from build123d import *

# Parameters (mm, degrees)
SKETCH_1_W          = 54
SKETCH_1_H          = 15
SKETCH_1_R          = 2.75
EXTRUDE_1_DEPTH     = 6
SKETCH_2_W          = 15
SKETCH_2_H          = 35
EXTRUDE_2_DEPTH     = 7.5
SKETCH_3_R          = 2.25
CUT_EXTRUDE_1_DEPTH = 15
CHAMFER_1_SIZE      = 2
FILLET_1_R          = 1


with BuildPart() as part:
    # 草图1 → 凸台-拉伸1 (new body)
    with BuildSketch(Plane(origin=(0, 0, 0), x_dir=(1, 0, 0), z_dir=(0, 1, 0))):
        Rectangle(SKETCH_1_W, SKETCH_1_H)
        with Locations(Location((-20, 0, 0), (0, 0, 270))):
            Circle(SKETCH_1_R, mode=Mode.SUBTRACT)
        with Locations(Location((20, 0, 0), (0, 0, 270))):
            Circle(SKETCH_1_R, mode=Mode.SUBTRACT)
    extrude(amount=EXTRUDE_1_DEPTH)

    # 草图2 → 凸台-拉伸2 (add, symmetric)
    with BuildSketch(Plane.XY):
        with Locations((0, 23.5)):
            Rectangle(SKETCH_2_W, SKETCH_2_H)
    extrude(amount=EXTRUDE_2_DEPTH, both=True)

    # 草图3 → 切除-拉伸1 (cut)
    with BuildSketch(Plane.ZY.offset(7.5)):
        with Locations(Location((0, 11, 0), (0, 0, 270))):
            Circle(SKETCH_3_R)
        with Locations(Location((0, 37, 0), (0, 0, 270))):
            Circle(SKETCH_3_R)
    extrude(amount=-CUT_EXTRUDE_1_DEPTH, mode=Mode.SUBTRACT)

    # 倒角1
    chamfer_1_edges = [part.edges().sort_by_distance(p)[0] for p in [
        (7.5, 6, 0),
        (-7.5, 6, 0),
    ]]
    chamfer(chamfer_1_edges, length=CHAMFER_1_SIZE)

    # 圆角1
    fillet_1_edges = [part.edges().sort_by_distance(p)[0] for p in [
        (-27, 6, 0),
        (-18.25, 6, 7.5),
        (0, 41, -7.5),
        (7.5, 41, 0),
        (-7.5, 24.5, -7.5),
        (-7.5, 41, 0),
        (0, 41, 7.5),
        (-7.5, 24.5, 7.5),
        (7.5, 24.5, -7.5),
        (7.5, 24.5, 7.5),
        (18.25, 6, 7.5),
        (-18.25, 6, -7.5),
        (27, 6, 0),
        (0, 0, 7.5),
        (8.5, 7, -7.5),
        (8.5, 7, 7.5),
        (-8.5, 7, -7.5),
        (-8.5, 7, 7.5),
        (-27, 0, 0),
        (0, 0, -7.5),
        (27, 0, 0),
        (27, 3, 7.5),
        (-27, 3, 7.5),
        (-27, 3, -7.5),
        (27, 3, -7.5),
        (18.25, 6, -7.5),
    ]]
    fillet(fillet_1_edges, radius=FILLET_1_R)


solid = part.part
Verification items for the finished model (mm, model axes). A direction names the side the tool comes from. Coordinates: 2 decimals unless noted, no trailing zeros. Loops run counter-clockwise (first coordinate to the right, second up) from the corner with the lowest first, then second, coordinate; pieces in that order, holes last. Notation, with made-up numbers: M -25,60 L -10,60 A19 ccw -10,66 Z; hole C -22,-34.5 d8. An arc over 180 degrees is marked long. One line per item, written item: value.
1. Set-up check for faces 5 (the flat face through (-7.5, 24, 0)), 6 (the cylindrical face through (-17.273, 2.958, -0.358)): record each of +Z, -Z, +X, -X, +Y, -Y from which the full face is reachable in a straight line by a thin tool's end or side.
Answers follow:
face 5: +Z, -Z, -X, +Y
face 6: +Y, -Y
2. Mould release check, pull along Y, two halves, no side actions. Record for faces 1 (the flat face through (16, 6, 0)), 2 (the cylindrical face through (-0.105, 13.248, 0.099)), 3 (the cylindrical face through (-0.11, 34.92, -0.86)), 4 (the flat face through (7.5, 24, 0)): pulls with the +Y half, pulls with the -Y half, needs draft (parallel to the pull), parting line crosses it, or undercut.
Answers follow:
face 1: pulls with the +Y half
face 2: undercut
face 3: undercut
face 4: needs draft
3. Section check C-C on z = 0. Give the number of separate pieces and of enclosed holes in the cut face, plus the area to 3 significant figures.
Answers follow:
separate pieces: 5
enclosed holes: 0
area: 651 mm^2
4. Section check B-B on y = 11. Record the cut outline in (x, z), plus the area to 3 significant figures.
Answers follow:
outline: M -7.5,-6.5 A1 ccw -6.5,-7.5 L 6.5,-7.5 A1 ccw 7.5,-6.5 L 7.5,-2.25 L -7.5,-2.25 Z; M -7.5,2.25 L 7.5,2.25 L 7.5,6.5 A1 ccw 6.5,7.5 L -6.5,7.5 A1 ccw -7.5,6.5 Z
area: 157 mm^2
5. Material ranges on line 1 along Z through (x, y) = (-1, 11); line 2 along X through (y, z) = (30, 4.5); line 3 along Y through (x, z) = (11, 4.5), recorded low to high. Write a range as from..to.
Answers follow:
line 1: -7.5..-2.25, 2.25..7.5
line 2: -7.5..7.5
line 3: 0..6
6. Gauge pin test, flat ends, axial feed: P1, Ø2, axis at x = 21, z = 3, coming from the +Y side; P2, Ø1.5, axis at y = 27.5, z = -2, coming from the +X side; P3, Ø4, axis at y = 18.5, z = -1, coming from the -X side. Record the tip position at first contact, or that the pin passes through.
Answers follow:
P1: y = 6
P2: x = 7.5
P3: x = -7.5
7. Section check A-A on x = -20. Record the cut outline in (y, z).
Answers follow:
outline: M 0,-6.5 A1 ccw 1,-7.5 L 5,-7.5 A1 ccw 6,-6.5 L 6,-2.75 L 0,-2.75 Z; M 0,2.75 L 6,2.75 L 6,6.5 A1 ccw 5,7.5 L 1,7.5 A1 ccw 0,6.5 Z
8. Section check D-D on y = 23.5. Record the cut outline in (x, z).
Answers follow:
outline: M -7.5,-6.5 A1 ccw -6.5,-7.5 L 6.5,-7.5 A1 ccw 7.5,-6.5 L 7.5,6.5 A1 ccw 6.5,7.5 L -6.5,7.5 A1 ccw -7.5,6.5 Z
